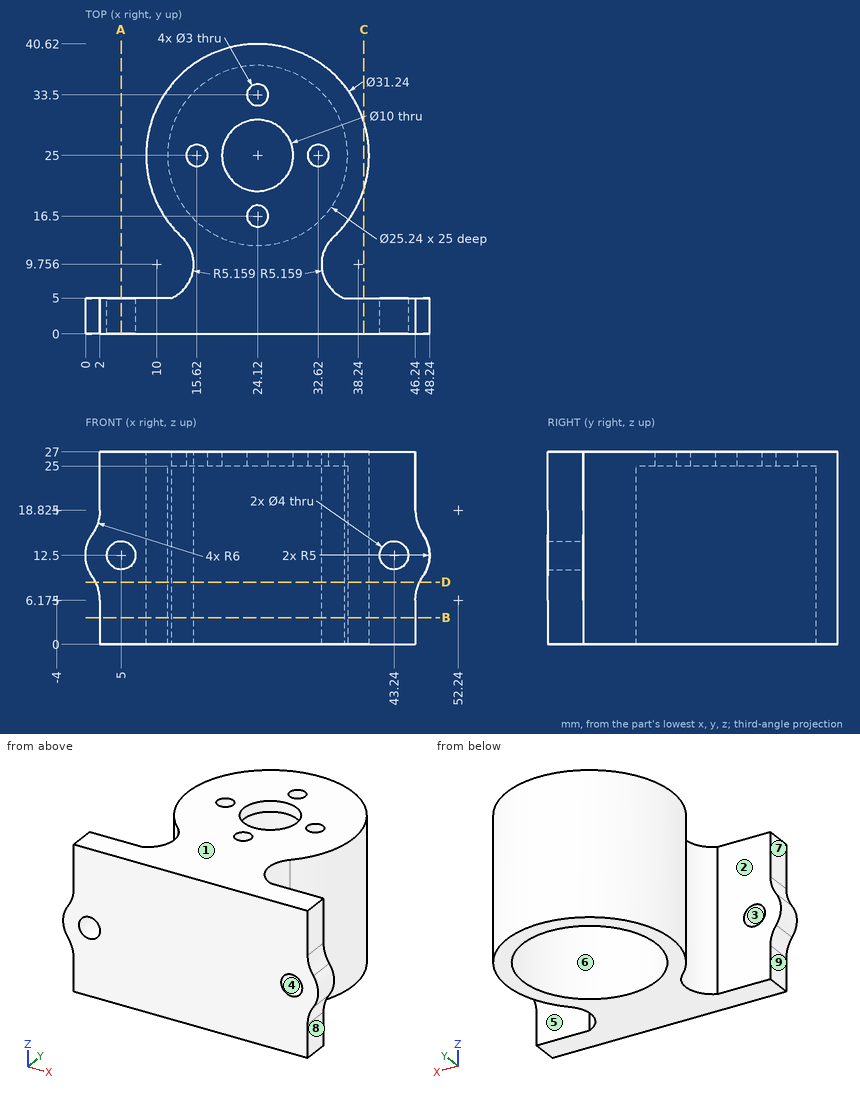
Job drawing, mm, ordinate dimensions from the low corner. One solid piece. A direction names the side the tool comes from. Give positions to 0.01 mm unless a question says otherwise; leave off trailing zeros. Loops run counter-clockwise (first coordinate to the right, second up) from the corner with the lowest first, then second, coordinate; pieces in that order, holes last. Notation, with made-up numbers: (2.5, 69.5) -> (23.5, 69.5) arc R6 ccw to (23.5, 73.5) -> close; hole circle Ø11 at (-29.75, 58). An arc over 180 degrees is marked (long way). Write each question's results on one line, items separated by ' | '. Start each with the question number.
Q1. Band-saw the part on A-A on x = 5. List the corners of the cut face in (y, z), plus the area to 3 significant figures.
Q2. Pull direction Z, two halves, no side cores. Call the marked faces 1, 2, 3 and 4: +Z half, -Z half, draft (parallel to the pull), parting line (faces both ways), or undercut.
Q3. Band-saw the part on D-D on z = 8.75. List the corners of the cut face in (x, y) (1 decimal).
Q4. Which spindle directions (+Z, -Z, +X, -X, +Y, -Y) get a long thin tool onto all of the face, cutting with end or side? Do the marked faces 5, 6, 7, 8 and 9. Say none if no direction does.
Q5. Band-saw the part on C-C on x = 39. List the corners of the cut face in (y, z).
Q6. Wall check: L1, parallel to X at y = 2.45, z = 12.5; L2, parallel to Y at x = 12.5, z = 4.25 (1 decimal); L3, parallel to Z at x = 15, y = 17.5. Give the ranges that are in metal, low to high.
Q7. Pin check, flat tips, straight feed: P1, Ø13, axis at x = 8.5, z = 19, coming from the +Y side; P2, Ø8, axis at y = 27.5, z = 19, coming from the -X side; P3, Ø12.5, axis at x = 28.5, y = 30, coming from the -Z side; P4, Ø13, axis at x = 24.12, y = 25, coming from the -Z side. Stop position of each tip, or through.
Q8. Band-saw the part on B-B on z = 3.75. List the corners of the cut face in (x, y) (1 decimal), plus the area to 3 significant figures.
Results are:
1) outline: (0, 0) -> (5, 0) -> (5, 10.5) -> (0, 10.5) -> close; (0, 14.5) -> (5, 14.5) -> (5, 27) -> (0, 27) -> close | area: 115 mm²
2) face 1: +Z half | face 2: draft | face 3: undercut | face 4: undercut
3) outline: (1.4, 0) -> (46.8, 0) -> (46.8, 5) -> (36.2, 5) arc R5.2 cw to (34.7, 13.5) arc R15.6 ccw (long way) to (13.5, 13.5) arc R5.2 cw to (12, 5) -> (1.4, 5) -> close; hole circle Ø25.2 at (24.1, 25)
4) face 5: +Z, -Z, +X | face 6: -Z | face 7: +Z, -X, +Y, -Y | face 8: -Z, +X, +Y, -Y | face 9: -Z, -X, +Y, -Y
5) outline: (0, 0) -> (5, 0) -> (5, 27) -> (0, 27) -> close; (20.25, 0) -> (29.75, 0) -> (29.75, 27) -> (20.25, 27) -> close
6) L1: x = 0 to 3, 7 to 41.24, 45.24 to 48.24 | L2: y = 0 to 5.2, 14.6 to 20.1, 29.9 to 35.4 | L3: z = 25 to 27
7) P1: stops at y = 37.68 | P2: stops at x = 8.5 | P3: stops at z = 0 | P4: stops at z = 25
8) outline: (2, 0) -> (46.2, 0) -> (46.2, 5) -> (36.2, 5) arc R5.2 cw to (34.7, 13.5) arc R15.6 ccw (long way) to (13.5, 13.5) arc R5.2 cw to (12, 5) -> (2, 5) -> close; hole circle Ø25.2 at (24.1, 25) | area: 592 mm²
